from build123d import *

# Parameters (mm, degrees)
F1_DEPTH = 10
F2_R     = 13.15
F3_DEPTH = 25
F5_DEPTH = 10.001
F6_R     = 3.5
F7_DEPTH = 10.001


with BuildPart() as f1:
    # F0 (on Front) → F1 (new body)
    with BuildSketch(Plane.XZ):
        with BuildLine():
            ThreePointArc((-49.6601038214, -17.9870707453), (-37.3753775975, -12.4844275463), (-32.3422225816, 0))
            ThreePointArc((-32.3422225816, 0), (-63.3090675656, 12.4844275463), (-49.6601038214, -17.9870707453))
        make_face()
        with BuildLine():
            Line((32.3422225816, 0), (-32.3422225816, 0))
            ThreePointArc((-32.3422225816, 0), (-37.3753775975, -12.4844275463), (-49.6601038214, -17.9870707453))
            Line((-49.6601038214, -17.9870707453), (50.3398953428, -17.9999998496))
            ThreePointArc((50.3398953428, -17.9999998496), (37.6134777436, -12.7270992316), (32.3422225816, 0))
        make_face()
        with BuildLine():
            ThreePointArc((68.3422225816, 0), (50.3422225816, 18), (32.3422225816, 0))
            ThreePointArc((32.3422225816, 0), (37.6134777436, -12.7270992316), (50.3398953428, -17.9999998496))
            ThreePointArc((50.3398953428, -17.9999998496), (63.0693218132, -12.7287448379), (68.3422225816, 0))
        make_face()
    extrude(amount=F1_DEPTH)

    # F2 (on face) → F3 (cut)
    with BuildSketch(Plane.XZ.offset(10)):
        with Locations((-50.3422225816, 0)):
            Circle(F2_R)
        with Locations((50.3422225816, 0)):
            Circle(F2_R)
    extrude(amount=-F3_DEPTH, mode=Mode.SUBTRACT)

    # F4 (on face) → F5 (cut, through all)
    with BuildSketch(Plane.XZ.offset(10)):
        with BuildLine():
            ThreePointArc((31.4967512046, -17.9975635998), (16.6000314606, -10.1934848087), (0, -7.5))
            Line((0, -7.5), (0, -17.993491352))
            Line((0, -17.993491352), (31.4967512046, -17.9975635998))
        make_face()
        with BuildLine():
            Line((0, -17.993491352), (0, -7.5))
            ThreePointArc((0, -7.5), (-16.5935917856, -10.1913389896), (-31.4858890741, -17.9894205085))
            Line((-31.4858890741, -17.9894205085), (0, -17.993491352))
        make_face()
    extrude(amount=-F5_DEPTH, mode=Mode.SUBTRACT)

    # F6 (on face) → F7 (cut, through all)
    with BuildSketch(Plane.XZ.offset(10)):
        with Locations((-30, -9.9896125538)):
            Circle(F6_R)
        with Locations((-20, -6)):
            Circle(F6_R)
        with Locations((19.0787840283, -6)):
            Circle(F6_R)
        with Locations((30, -9.9973700164)):
            Circle(F6_R)
    extrude(amount=-F7_DEPTH, mode=Mode.SUBTRACT)


solid = f1.part
Geometry check sheet. Reference: the model listing, model coordinates, mm. Give positions to 0.01 mm unless a question says otherwise; leave off trailing zeros. Loops run counter-clockwise (first coordinate to the right, second up) from the corner with the lowest first, then second, coordinate; pieces in that order, holes last. Notation, with made-up numbers: M 70.5,-13 L 97.5,-13 A31 ccw 97.5,18 Z; hole C 40,61.25 d3. An arc over 180 degrees is marked long. Write each question's results on one line, items separated by ' | '.
1) Section check D-D, the plane x = 17. Record the boundary of the cut face in (y, z).
Answers follow:
outline: M -10,-10.33 L 0,-10.33 L 0,-8.82 L -10,-8.82 Z; M -10,-3.18 L 0,-3.18 L 0,0 L -10,0 Z
2) Section check C-C, the plane y = -3.25. Record the boundary of the cut face in (x, z).
Answers follow:
outline: M -49.66,-17.99 L -31.49,-17.99 A52.5 cw 31.5,-18 L 50.34,-18 A18 ccw long 32.34,0 L -32.34,0 A18 ccw long Z; hole C -50.34,0 d26.3; hole C -30,-9.99 d7; hole C -20,-6 d7; hole C 19.08,-6 d7; hole C 30,-10 d7; hole C 50.34,0 d26.3
3) Section check B-B, the plane z = 6.5. Record the boundary of the cut face in (x, y), plus the area to 3 significant figures.
Answers follow:
outline: M -67.13,-10 L -61.77,-10 L -61.77,0 L -67.13,0 Z; M -38.91,-10 L -33.56,-10 L -33.56,0 L -38.91,0 Z; M 33.56,-10 L 38.91,-10 L 38.91,0 L 33.56,0 Z; M 61.77,-10 L 67.13,-10 L 67.13,0 L 61.77,0 Z | area: 214 mm2
4) Release check for a two-part mould opening along Z. For faces 1 (the face through (0, -5, 0)), 2 (the face through (0, -10, -3)), 3 (the face through (31.882, -5.07, -7.046)) record: +Z half, -Z half, draft (parallel to the pull), parting line (faces both ways), or undercut.
Answers follow:
face 1: +Z half | face 2: draft | face 3: undercut
5) Section check A-A, the plane x = -20. Record the boundary of the cut face in (y, z).
Answers follow:
outline: M -10,-11.46 L 0,-11.46 L 0,-9.5 L -10,-9.5 Z; M -10,-2.5 L 0,-2.5 L 0,0 L -10,0 Z
6) Thickness scan on line 1 (X direction, y = -1.75, z = 7); line 2 (X direction, y = -8, z = 4); line 3 (X direction, y = -5, z = -1). Record the ranges inside material, lowest first.
Answers follow:
line 1: -66.93 to -61.47, -39.21 to -33.76, 33.76 to 39.21, 61.47 to 66.93 | line 2: -67.89 to -62.87, -37.82 to -32.79, 32.79 to 37.82, 62.87 to 67.89 | line 3: -68.31 to -63.45, -37.23 to 37.23, 63.45 to 68.31
7) Gauge pin test, flat ends, axial feed: pin 1 (4 mm diameter, centred on x = -42.5, y = -6.5, fed in from -Z); pin 2 (1 mm diameter, centred on y = -7.5, z = 1, fed in from +X); pin 3 (3 mm diameter, centred on x = -7.5, y = -3.5, fed in from +Z). Record the tip position at first contact, or that the pin passes through.
Answers follow:
pin 1: z = -17.99 | pin 2: x = 68.34 | pin 3: z = 0
